```python
from build123d import *

# Parameters (mm, degrees)
SKETCH1_W           = 30
SKETCH1_H           = 100
BOSS_EXTRUDE1_DEPTH = 10
SKETCH2_R           = 5
CUT_EXTRUDE1_DEPTH  = 10
FILLET1_R           = 10
FILLET2_R           = 10


with BuildPart() as part:
    # Sketch1 → Boss-Extrude1 (new body)
    with BuildSketch(Plane(origin=(0, 0, 0), x_dir=(1, 0, 0), z_dir=(0, 1, 0))):
        Rectangle(SKETCH1_W, SKETCH1_H)
    extrude(amount=BOSS_EXTRUDE1_DEPTH)

    # Sketch2 → Cut-Extrude1 (cut)
    with BuildSketch(Plane(origin=(0, 10, 0), x_dir=(1, 0, 0), z_dir=(0, 1, 0))):
        with Locations(Location((0, 40, 0), (0, 0, 270))):
            Circle(SKETCH2_R)
        with Locations(Location((0, -40, 0), (0, 0, 270))):
            Circle(SKETCH2_R)
    extrude(amount=-CUT_EXTRUDE1_DEPTH, mode=Mode.SUBTRACT)

    # Fillet1
    fillet1_edges = [part.edges().sort_by_distance(p)[0] for p in [
        (15, 5, 50),
        (-15, 5, 50),
    ]]
    fillet(fillet1_edges, radius=FILLET1_R)

    # Fillet2
    fillet2_edges = [part.edges().sort_by_distance(p)[0] for p in [
        (-15, 5, -50),
        (15, 5, -50),
    ]]
    fillet(fillet2_edges, radius=FILLET2_R)


solid = part.part
```
The model under review builds one solid part; all positions refer to its coordinate system, in mm. Coordinates: 2 decimals unless noted, no trailing zeros. Order: outer loops, then holes, each group sorted by start corner. A loop starts at its lowest first (then second) coordinate and runs counter-clockwise, first axis right, second up. Notation, with made-up numbers: M 48.25,5 L 96.25,5 A28 ccw 96.25,38 Z; hole C 43,-36.75 d8. An arc over 180 degrees is marked long. One line per question, with ' | ' between items.
(1) The part is to be moulded in two halves that separate along X. For faces 1 (the face through (0, 5, -45)), 2 (the face through (11.99, 5.07, 47.15)), 3 (the face through (0, 0, -1)), say which applies: +X half, -X half, draft (parallel to the pull), parting line (faces both ways), or undercut.
Geometry results:
face 1: undercut | face 2: +X half | face 3: draft
(2) Add section C-C, the plane y = 6. Write out the cut boundary in (x, z).
Geometry results:
outline: M -15,-40 A10 ccw -5,-50 L 5,-50 A10 ccw 15,-40 L 15,40 A10 ccw 5,50 L -5,50 A10 ccw -15,40 Z; hole C 0,-40 d10; hole C 0,40 d10
(3) Add section B-B, the plane z = 36. Write out the cut boundary in (x, y).
Geometry results:
outline: M -15,0 L -3,0 L -3,10 L -15,10 Z; M 3,0 L 15,0 L 15,10 L 3,10 Z
(4) For probe 1 along X at (y, z) = (4.5, -40); probe 2 along Z at (x, y) = (-1, 6.75); probe 3 along Z at (x, y) = (-2, 8.25), list the stretches that pass through material, from the lowest coordinate up. Write a range as from..to.
Geometry results:
probe 1: x = -15..-5, 5..15 | probe 2: z = -50..-44.9, -35.1..35.1, 44.9..50 | probe 3: z = -50..-44.58, -35.42..35.42, 44.58..50
(5) Add section A-A, the plane x = 0. Write out the cut boundary in (y, z).
Geometry results:
outline: M 0,-50 L 10,-50 L 10,-45 L 0,-45 Z; M 0,-35 L 10,-35 L 10,35 L 0,35 Z; M 0,45 L 10,45 L 10,50 L 0,50 Z
(6) Add section D-D, the plane x = 9. Write out the cut boundary in (y, z).
Geometry results:
outline: M 0,-49.17 L 10,-49.17 L 10,49.17 L 0,49.17 Z
(7) Insertion check: pin 1 (4 mm diameter, centred on x = 9, y = 6, fed in from +Z); pin 2 (6 mm diameter, centred on x = 0, z = -40, fed in from -Y). Each pin has a flat end and moves straight along its axis. Give the tip position at first contact, or say it passes through.
Geometry results:
pin 1: stops at z = 49.8 | pin 2: passes through
